Verification items for the finished model (mm, model axes). A direction names the side the tool comes from. Give positions to 0.01 mm unless a question says otherwise; leave off trailing zeros. Write each loop counter-clockwise with the first axis right and the second up, starting at its lowest first coordinate (ties: lowest second). Pieces come first, ordered by that corner, then holes. Notation, with made-up numbers: M 27.5,-12.75 L 39.5,-12.75 A17 ccw 39.5,-5.75 Z; hole C -32.5,6 d7. An arc over 180 degrees is marked long. Answer as a JSON object with one key per item and string values.
Autodesk Fusion 360 part; units mm, degrees
sketch "Sketch1" plane through (0, 0, 0) normal (0, 0, 1) x (1, 0, 0)
  circle A0 centre (-19.9657, -62) radius 2
  line L0 (6.2753, -74) -> (14.4853, -74) construction
  line L1 (0.2753, -24) -> (-39.2258, -24)
  line L2 (6.2753, -74) -> (0.2753, -68)
  line L3 (-39.2258, -80) -> (-39.2258, -52)
  circle A1 centre (3, -77) radius 1.75
  circle A2 centre (-43, -77) radius 1.75
  line L4 (6.2753, -80) -> (6.2753, -74)
  line L5 (0.2753, -80) -> (6.2753, -80)
  line L6 (0.2753, -52) -> (0.2753, -24)
  line L7 (-46, -80) -> (-46, -74)
  line L8 (-39.2258, -80) -> (-46, -80)
  circle A3 centre (3.2753, -27) radius 1.75
  line L9 (-39.2258, -24) -> (-45.2258, -24)
  line L10 (6.2753, -30) -> (0.2753, -36)
  line L11 (-45.2258, -24) -> (-45.2258, -30)
  line L12 (0.2753, -24) -> (6.2753, -24)
  line L13 (-45.2258, -30) -> (-37.5147, -30) construction
  line L14 (-45.2258, -30) -> (-39.2258, -36)
  circle A4 centre (-19.9982, -42) radius 2
  line L15 (6.2753, -24) -> (6.2753, -30)
  line L16 (0.2753, -52) -> (0.2753, -80)
  line L17 (-19.9982, -42) -> (-19.9657, -62)
  line L18 (0.2753, -80) -> (-39.2258, -80)
  line L19 (-46, -74) -> (-39.2258, -67.2258)
  line L20 (-39.2258, -52) -> (0.2753, -52)
  line L21 (-39.2258, -24) -> (-39.2258, -52)
  circle A5 centre (-42.2258, -27) radius 1.75
  point P0 (0.2753, -24)
  dimension "d16" = 4
  dimension "d20" = 20
  dimension "d21" = 4
  dimension "d30" = 6
  dimension "d31" = 6
  dimension "d32" = 135
  dimension "d33" = 3.5
  dimension "d34" = 6
  dimension "d35" = 6
  dimension "d36" = 3.5
  dimension "d37" = 6
  dimension "d38" = 6
  dimension "d39" = 45
  dimension "d41" = 135
  dimension "d42" = 3.5
  dimension "d54" = 10
  dimension "d52" = 56
  dimension "d53" = 3.5
  dimension "d55" = 3
  dimension "d56" = 28
extrude "Extrude1" add sketch "Sketch1" along normal blind 5 contours L3 L16 L18 L20 | L1 L6 L20 L21
extrude "Extrude2" add sketch "Sketch1" along normal blind 5 contours L3 L7 L8 L19 | L9 L11 L14 L21 | L6 L10 L12 L15 | L2 L4 L5 L16
sketch "Sketch2" plane through (0, 0, 5) normal (0, 0, 1) x (-1, 0, 0)
  circle A0 centre (-3, 77) radius 1.75
  circle A1 centre (43, 77) radius 1.75
  circle A2 centre (-3.2753, 27) radius 1.75
  circle A3 centre (19.9982, 42) radius 2
  circle A4 centre (19.9657, 62) radius 2
  line L0 (-0.2753, 68) -> (-0.2753, 36)
  line L1 (-0.2753, 36) -> (-6.2753, 30)
  line L2 (-6.2753, 30) -> (-6.2753, 24)
  line L3 (-6.2753, 24) -> (45.2258, 24)
  line L4 (45.2258, 24) -> (45.2258, 30)
  line L5 (45.2258, 30) -> (39.2258, 36)
  line L6 (39.2258, 36) -> (39.2258, 67.2258)
  line L7 (39.2258, 67.2258) -> (46, 74)
  line L8 (46, 74) -> (46, 80)
  line L9 (46, 80) -> (-6.2753, 80)
  line L10 (-6.2753, 80) -> (-6.2753, 74)
  line L11 (-6.2753, 74) -> (-0.2753, 68)
  line L12 (4.7247, 24) -> (4.7247, 104)
  line L13 (-0.2753, 52) -> (-0.2753, 24)
  line L14 (-0.2753, 24) -> (-0.2753, 80)
  dimension "d25" = 80
  dimension "d26" = 5
extrude "Extrude3" add sketch "Sketch2" along normal blind 15.5 contours L0 L3 L9 L12 L13 L14
sketch "Sketch3" plane through (0, 0, 20.5) normal (0, 0, 1) x (-1, 0, 0)
  line L0 (4.7247, 24) -> (4.7247, 80)
  line L1 (4.7247, 80) -> (-0.2753, 80)
  line L2 (-0.2753, 80) -> (-0.2753, 24)
  line L3 (-0.2753, 24) -> (4.7247, 24)
  line L4 (39.1553, 24.0265) -> (-0.2753, 24.0265)
  line L5 (-0.2753, 80) -> (39.1553, 80)
  line L6 (39.1553, 80) -> (39.1553, 24.0265)
extrude "Extrude4" add sketch "Sketch3" along normal blind 5 contours L0 L1 L2 L4 L5
extrude "Extrude5" add sketch "Sketch3" along normal blind 5 contours L0 L4 L5 L6
hole "Hole1" at (-19.8305, -62, 0) direction (0, 0, 1) diameter 4 depth 31 tip angle 118
hole "Hole2" at (-19.863, -42, 0) direction (0, 0, 1) diameter 4 depth 30 tip angle 118
hole "Hole3" at (-42.2258, -27, 0) direction (0, 0, 1) diameter 4 depth 11 tip angle 118
equation "d54 = d20 / 2"
equation "d56 = d52 / 2"
1) Release check for a two-part mould opening along X. For faces 4 (the face through (3.317, -32.958, 2.465)), 5 (the face through (-4.725, -52, 13)), 6 (the face through (-22, -42, 2)) record: pulls with the +X half, pulls with the -X half, needs draft (parallel to the pull), parting line crosses it, or undercut.
Completed:
{"face 4": "pulls with the +X half", "face 5": "pulls with the -X half", "face 6": "undercut"}
2) Section check D-D on y = -42. Record the boundary of the cut face in (x, z).
Completed:
{"outline": "M -39.23,0 L -22,0 L -22,5 L -39.23,5 Z; M -39.16,20.5 L -21.86,20.5 L -21.86,25.5 L -39.16,25.5 Z; M -17.86,0 L 0.28,0 L 0.28,25.5 L -17.86,25.5 L -17.86,20.5 L -4.72,20.5 L -4.72,5 L -17.86,5 Z"}
3) Section check B-B on y = -27. Record the boundary of the cut face in (x, z).
Completed:
{"outline": "M -45.23,0 L -44.23,0 L -44.23,5 L -45.23,5 Z; M -40.23,0 L 1.53,0 L 1.53,5 L 0.28,5 L 0.28,25.5 L -39.16,25.5 L -39.16,20.5 L -4.72,20.5 L -4.72,5 L -40.23,5 Z; M 5.03,0 L 6.28,0 L 6.28,5 L 5.03,5 Z"}
4) Go/stop test with flat-tipped pins: pin 1 (10 mm diameter, centred on y = -38, z = 14, fed in from -X); pin 2 (5.5 mm diameter, centred on x = -14, z = 23.5, fed in from +Y); pin 3 (5.5 mm diameter, centred on y = -50, z = 3.5, fed in from -X). Record where each tip stops, or that it passes through.
Completed:
{"pin 1": "stops at x = -4.72", "pin 2": "stops at y = -24.03", "pin 3": "stops at x = -39.23"}
5) Section check A-A on x = -17. Record the boundary of the cut face in (y, z).
Completed:
{"outline": "M -80,0 L -24,0 L -24,5 L -80,5 Z; M -80,20.5 L -24.03,20.5 L -24.03,25.5 L -80,25.5 Z"}
6) Thickness scan on L1, parallel to X at y = -77, z = 3.65; L2, parallel to Z at x = -14, y = -56; L3, parallel to Y at x = 3, z = 1.95. Record the ranges inside material, lowest first.
Completed:
{"L1": "x = -46 to -44.75, -41.25 to 1.25, 4.75 to 6.28", "L2": "z = 0 to 5, 20.5 to 25.5", "L3": "y = -80 to -78.75, -75.25 to -70.72, -33.28 to -28.73, -25.27 to -24"}
7) Section check C-C on x = 3. Record the boundary of the cut face in (y, z).
Completed:
{"outline": "M -80,0 L -78.75,0 L -78.75,5 L -80,5 Z; M -75.25,0 L -70.72,0 L -70.72,5 L -75.25,5 Z; M -33.28,0 L -28.73,0 L -28.73,5 L -33.28,5 Z; M -25.27,0 L -24,0 L -24,5 L -25.27,5 Z"}
8) Access from +Z, -Z, +X, -X, +Y, -Y to the whole of each face (thin tool, end or side, straight path). Record for faces 1 (the face through (-45.226, -27, 2)), 2 (the face through (-39.226, -52, 2)), 3 (the face through (2, -29, 5)).
Completed:
{"face 1": "+Z, -Z, -X, +Y", "face 2": "+Z, -Z, -X", "face 3": "+Z, +X, +Y, -Y"}
